Design review of the part built by this model. Coordinates are the model's own, in mm. Face numbers are marked on the shaded views. A direction names the side the tool comes from. Coordinates: 2 decimals unless noted, no trailing zeros. Write each loop counter-clockwise with the first axis right and the second up, starting at its lowest first coordinate (ties: lowest second). Pieces come first, ordered by that corner, then holes.
Q1. Take a section at D-D (x = 95.5). Give the boundary of the cut face in (y, z), and give its area (3 significant figures).
Q2. Take a section at B-B (z = -12). Give the boundary of the cut face in (x, y).
Q3. Machinability: for the marked faces 3, 4 and 5, which of the approach directions +Z, -Z, +X, -X, +Y, -Y give a long, thin tool a straight path to every point of the face, cutting with its end or side? Answer none if there is none.
Q4. Mouldability with a two-part tool opening along X and no side actions: class the marked faces 1 and 2 as pulls with the +X half, pulls with the -X half, needs draft (parallel to the pull), parting line crosses it, or undercut.
Q5. For probe 1 along Y at (x, z) = (62.5, -24.25); probe 2 along X at (y, z) = (35, -17.5); probe 3 along Z at (x, y) = (52, 8.5), list the stretches that pass through material, from the lowest coordinate up.
Q6. Insertion check: pin 1 (11 mm diameter, centred on x = 69.5, z = -16.5, fed in from +Y); pin 2 (5 mm diameter, centred on x = 114, y = 56, fed in from +Z); pin 3 (2 mm diameter, centred on x = 102, y = 57.5, fed in from +Z). Each pin has a flat end and moves straight along its axis. Give the tip position at first contact, or say it passes through.
Q7. Take a section at A-A (x = 35). Give the boundary of the cut face in (y, z).
Q8. Take a section at C-C (y = 24). Give the boundary of the cut face in (x, z).
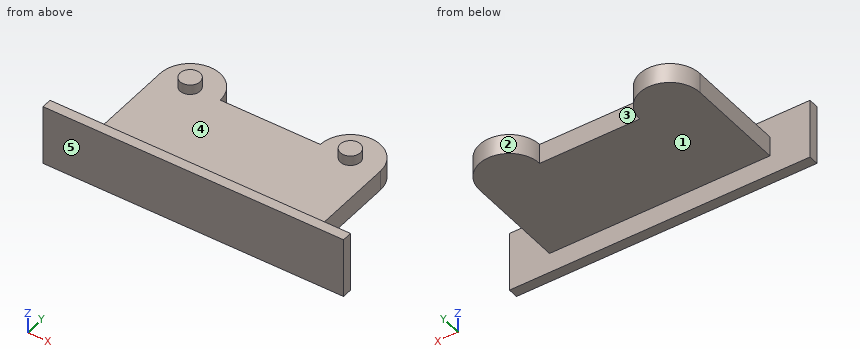
Autodesk Inventor part; units mm, degrees
ref_plane "YZ Plane" through (0, 0, 0) normal (1, 0, 0) x (0, 1, 0)
ref_plane "XZ Plane" through (0, 0, 0) normal (0, 1, 0) x (-1, 0, 0)
ref_plane "XY Plane" through (0, 0, 0) normal (0, 0, 1) x (1, 0, 0)
sketch "Эскиз1" plane through (0, 0, 0) normal (0, 1, 0) x (-1, 0, 0)
  line L0 (0, 0) -> (-150, 0)
  line L1 (-150, 0) -> (-150, -30)
  line L2 (-150, -30) -> (0, -30)
  line L3 (0, -30) -> (0, 0)
  dimension "d0" = 150
  dimension "d1" = 30
extrude "Выдавливание1" add sketch "Эскиз1" along normal blind 5
sketch "Эскиз3" plane through (0, 5, 0) normal (0, 1, 0) x (1, 0, 0)
  line L0 (20, 20) -> (130, 20)
  line L1 (130, 20) -> (130, 10)
  line L2 (130, 10) -> (20, 10)
  line L3 (20, 10) -> (20, 20)
  line L4 (150, 30) -> (0, 30)
  line L5 (0, 0) -> (150, 0)
  line L6 (0, 30) -> (0, 0)
  line L7 (150, 0) -> (150, 30)
  dimension "d8" = 10
  dimension "d9" = 10
  dimension "d10" = 20
  dimension "d11" = 20
extrude "Выдавливание3" add sketch "Эскиз3" along normal blind 50 contours L0 L1 L2 L3
sketch "Эскиз4" plane through (20, 5, -10) normal (0, 0, 1) x (1, 0, 0)
  arc A0 (30, 50) -> (0, 50) centre (15, 50) ccw
  line L0 (0, 50) -> (110, 50)
  line L1 (0, 0) -> (0, 50)
  line L2 (55, 50) -> (55, 234.7508)
  arc A1 (110, 50) -> (80, 50) centre (95, 50) ccw
  point P0 (-20, -5)
  dimension "d14" = 30
extrude "Выдавливание4" add sketch "Эскиз4" against normal up to surface (10 mm away)
sketch "Эскиз5" plane through (20, 5, -10) normal (0, 0, 1) x (1, 0, 0)
  arc A0 (30, 50) -> (0, 50) centre (15, 50) ccw
  arc A1 (110, 50) -> (80, 50) centre (95, 50) ccw
  circle A2 centre (15, 50) radius 5
  circle A3 centre (95, 50) radius 5
  point P0 (-20, -5)
  point P1 (55, 199.7494)
  dimension "d24" = 10
  dimension "d25" = 10
extrude "Выдавливание5" add sketch "Эскиз5" along normal blind 5
properties part number "Base"
Response:
1. outline: (0, -30) - (5, -30) - (5, -20) - (55, -20) - (55, -10) - (5, -10) - (5, 0) - (0, 0) - close
1. area: 650 mm2
2. outline: (0, 0) - (150, 0) - (150, 5) - (130, 5) - (130, 55) arc R15 ccw to (100, 55) - (50, 55) arc R15 ccw to (20, 55) - (20, 5) - (0, 5) - close
3. face 3: +Z, -Z, +Y
3. face 4: +Z
3. face 5: +Z, -Z, +X, -X, -Y
4. face 1: needs draft
4. face 2: undercut
5. probe 1: y = 0 to 5
5. probe 2: x = 20 to 130
5. probe 3: z = -20 to -10
6. pin 1: stops at y = 55
6. pin 2: stops at z = -5
6. pin 3: stops at z = -10
7. outline: (0, -30) - (5, -30) - (5, -20) - (70, -20) - (70, -10) - (60, -10) - (60, -5) - (50, -5) - (50, -10) - (5, -10) - (5, 0) - (0, 0) - close
8. outline: (20, -20) - (130, -20) - (130, -10) - (20, -10) - close
